Check sheet for the drawn part. Datum: minimum x, y, z corner. Units: mm. Give positions to 0.01 mm unless a question says otherwise; leave off trailing zeros. Order: outer loops, then holes, each group sorted by start corner. A loop starts at its lowest first (then second) coordinate and runs counter-clockwise, first axis right, second up.
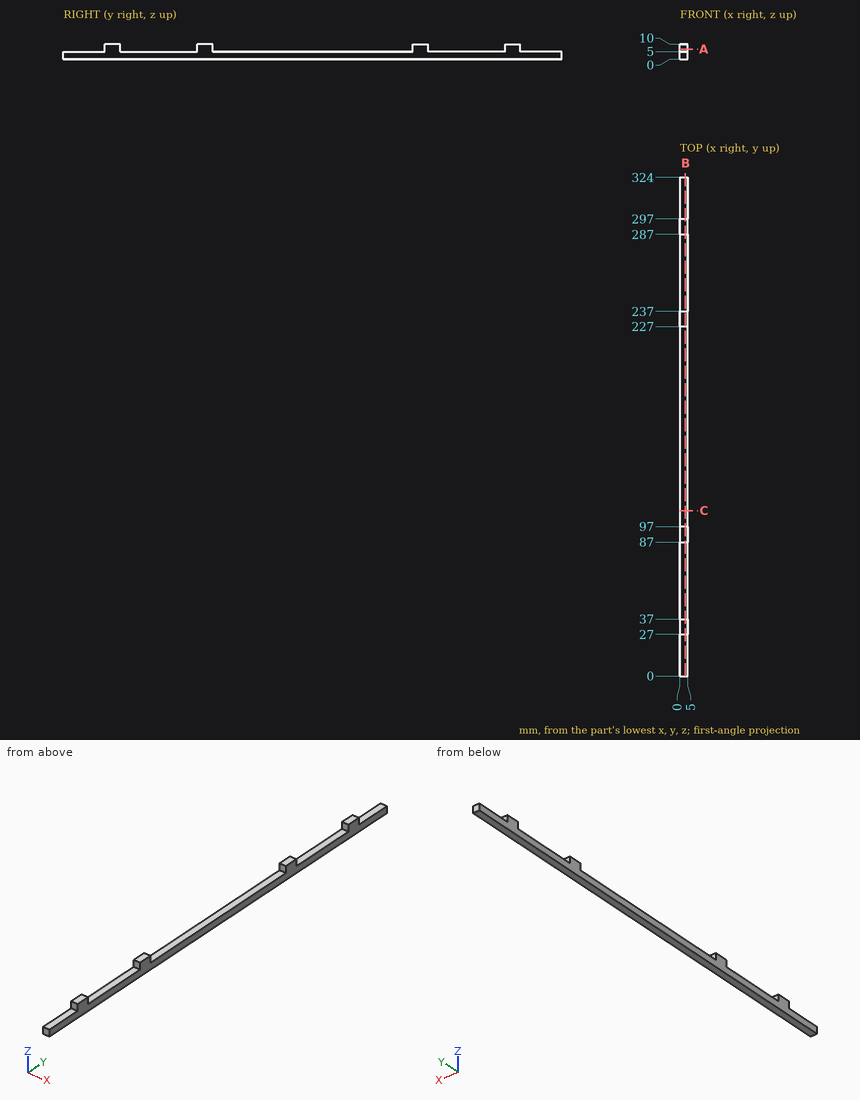
Item 1: Gauge pin test, flat ends, axial feed: pin 1 (1.5 mm diameter, centred on x = 2.5, z = 7, fed in from -Y); pin 2 (1.5 mm diameter, centred on x = 1.5, z = 7, fed in from +Y); pin 3 (2.5 mm diameter, centred on x = 1.5, y = 272, fed in from +Z). Record the tip position at first contact, or that the pin passes through.
Reported:
pin 1: stops at y = 27
pin 2: stops at y = 297
pin 3: stops at z = 5
Item 2: Sectioned sample at B-B (x = 3.6). Enter the section's corners in (y, z), and give its area (3 significant figures).
Reported:
outline: (0, 0) - (324, 0) - (324, 5) - (297, 5) - (297, 10) - (287, 10) - (287, 5) - (237, 5) - (237, 10) - (227, 10) - (227, 5) - (97, 5) - (97, 10) - (87, 10) - (87, 5) - (37, 5) - (37, 10) - (27, 10) - (27, 5) - (0, 5) - close
area: 1,820 mm2
Item 3: Scan lines: L1, parallel to Y at x = 2.15, z = 5.75; L2, parallel to Z at x = 0.5, y = 57.5. Record each from-to range of solid material in increasing order.
Reported:
L1: y = 27 to 37, 87 to 97, 227 to 237, 287 to 297
L2: z = 0 to 5
Item 4: Sectioned sample at A-A (z = 6.75). Enter the section's corners in (x, y).
Reported:
outline: (0, 27) - (5, 27) - (5, 37) - (0, 37) - close; (0, 87) - (5, 87) - (5, 97) - (0, 97) - close; (0, 227) - (5, 227) - (5, 237) - (0, 237) - close; (0, 287) - (5, 287) - (5, 297) - (0, 297) - close
Item 5: Sectioned sample at C-C (y = 107.5). Enter the section's corners in (x, z), and give its area (3 significant figures).
Reported:
outline: (0, 0) - (5, 0) - (5, 5) - (0, 5) - close
area: 25.0 mm2
